Geometry check sheet. Reference: the model listing, model coordinates, mm. A direction names the side the tool comes from. Coordinates: 2 decimals unless noted, no trailing zeros. Write each loop counter-clockwise with the first axis right and the second up, starting at its lowest first coordinate (ties: lowest second). Pieces come first, ordered by that corner, then holes. Notation, with made-up numbers: (-11, 40) -> (-7, 40) arc R26 cw to (-7, 56) -> close; hole circle Ø5 at (-2, -30). An arc over 180 degrees is marked (long way). Answer in a Markdown table with one row per item. Add a question column.
1. Mould release check, pull along Z, two halves, no side actions. Record for faces 1 (the flat face through (6, 28.05, 35)), 2 (the flat face through (2, 14, 26)), 3 (the flat face through (8.9, 5.8, -18.2)): pulls with the +Z half, pulls with the -Z half, needs draft (parallel to the pull), parting line crosses it, or undercut.
2. Set-up check for faces 4 (the flat face through (6, 24.5, 35)), 5 (the flat face through (0, 10, 0)), 6 (the flat face through (6, 31, -46)), 7 (the cylindrical face through (5.9, 31.2, 40.5)), 8 (the flat face through (7.67, 8.09, 18.41)): record each of +Z, -Z, +X, -X, +Y, -Y from which the full face is reachable in a straight line by a thin tool's end or side.
3. Depth check by flat-ended pin: P1, Ø0.8, axis at x = 5.5, z = -34.5, coming from the -Y side; P2, Ø5.5, axis at y = 10, z = -5, coming from the +X side; P3, Ø6, axis at y = 28, z = -17, coming from the +X side. Enter the tip coordinate at first touch or a pass-through.
4. Cross-section at B-B on y = 21.5. Record the cut outline in (x, z), and give its area (3 significant figures).
5. Scan lines: L1, parallel to Z at x = 8, y = 9; L2, parallel to Y at x = 6.5, z = 37; L3, parallel to X at y = 19, z = -5.5. Record each from-to range of solid material in increasing order. Write a range as from..to.
```python
from build123d import *

# Parameters (mm, degrees)
BOSS_EXTRUDE1_DEPTH = 46
CUT_EXTRUDE1_REACH  = 62.101
SKETCH2_W           = 20
SKETCH2_H           = 24.5
FILLET1_R           = 2
FILLET2_R           = 4
CUT_EXTRUDE2_REACH  = 62.101
SKETCH4_R           = 4.3
BOSS_EXTRUDE2_DEPTH = 1.3
SKETCH5_R           = 4.25
BOSS_EXTRUDE3_DEPTH = 5
CHAMFER1_SIZE       = 0.3
CUT_EXTRUDE3_DEPTH  = 2.5


with BuildPart() as part:
    # Sketch1 → Boss-Extrude1 (new, symmetric)
    with BuildSketch(Plane.XY):
        with BuildLine():
            Line((0, 0), (2.6, 0))
            Line((2.6, 0), (2.6, 19))
            ThreePointArc((2.6, 19), (2.892893219, 19.707106781), (3.6, 20))
            Line((3.6, 20), (3.618034897, 20))
            ThreePointArc((3.618034897, 20), (6.16361931, 21.054415588), (7.218034897, 23.6))
            Line((7.218034897, 23.6), (7.218034897, 38))
            Line((7.218034897, 38), (4.618034897, 38))
            Line((4.618034897, 38), (4.618034897, 23.6))
            ThreePointArc((4.618034897, 23.6), (4.325141678, 22.892893219), (3.618034897, 22.6))
            Line((3.618034897, 22.6), (3.6, 22.6))
            ThreePointArc((3.6, 22.6), (1.054415588, 21.545584412), (0, 19))
            Line((0, 19), (0, 0))
        make_face()
    extrude(amount=BOSS_EXTRUDE1_DEPTH, both=True)

    # Sketch2 → Cut-Extrude1 (cut, up to next)
    with BuildSketch(Plane(origin=(7.218034897, 0, 0), x_dir=(0, 0, -1), z_dir=(1, 0, 0)), mode=Mode.PRIVATE) as cut_extrude1_sk1:
        with Locations((-36, 12.25)):
            Rectangle(SKETCH2_W, SKETCH2_H)
    cut_extrude1_tool1 = extrude(cut_extrude1_sk1.sketch, amount=-CUT_EXTRUDE1_REACH, mode=Mode.PRIVATE) & part.part
    # Sketch2 → Cut-Extrude1 (cut, up to next)
    with BuildSketch(Plane(origin=(7.218034897, 0, 0), x_dir=(0, 0, -1), z_dir=(1, 0, 0)), mode=Mode.PRIVATE) as cut_extrude1_sk2:
        with Locations((36, 12.25)):
            Rectangle(SKETCH2_W, SKETCH2_H)
    cut_extrude1_tool2 = extrude(cut_extrude1_sk2.sketch, amount=-CUT_EXTRUDE1_REACH, mode=Mode.PRIVATE) & part.part
    add(cut_extrude1_tool1.solids().sort_by_distance((7.218035, 12.25, 36))[0], mode=Mode.SUBTRACT)
    add(cut_extrude1_tool2.solids().sort_by_distance((7.218035, 12.25, -36))[0], mode=Mode.SUBTRACT)

    # Fillet1
    fillet1_edges = [part.edges().sort_by_distance(p)[0] for p in [
        (5.918034897, 38, -46),
        (5.918034897, 38, 46),
        (5.918034897, 24.5, 46),
        (5.918034897, 24.5, -46),
    ]]
    fillet(fillet1_edges, radius=FILLET1_R)

    # Fillet2
    fillet2_edges = [part.edges().sort_by_distance(p)[0] for p in [
        (1.3, 0, 26),
        (1.3, 0, -26),
    ]]
    fillet(fillet2_edges, radius=FILLET2_R)

    # Sketch3 → Cut-Extrude2 (cut, up to next)
    with BuildSketch(Plane(origin=(7.218034897, 0, 0), x_dir=(0, 0, -1), z_dir=(1, 0, 0)), mode=Mode.PRIVATE) as cut_extrude2_sk1:
        with BuildLine():
            Line((-37.25, 34.55), (-33.25, 34.55))
            ThreePointArc((-33.25, 34.55), (-30, 31.3), (-33.25, 28.05))
            Line((-33.25, 28.05), (-37.25, 28.05))
            ThreePointArc((-37.25, 28.05), (-40.5, 31.3), (-37.25, 34.55))
        make_face()
    cut_extrude2_tool1 = extrude(cut_extrude2_sk1.sketch, amount=-CUT_EXTRUDE2_REACH, mode=Mode.PRIVATE) & part.part
    # Sketch3 → Cut-Extrude2 (cut, up to next)
    with BuildSketch(Plane(origin=(7.218034897, 0, 0), x_dir=(0, 0, -1), z_dir=(1, 0, 0)), mode=Mode.PRIVATE) as cut_extrude2_sk2:
        with BuildLine():
            Line((37.25, 34.55), (33.25, 34.55))
            ThreePointArc((33.25, 34.55), (30, 31.3), (33.25, 28.05))
            Line((33.25, 28.05), (37.25, 28.05))
            ThreePointArc((37.25, 28.05), (40.5, 31.3), (37.25, 34.55))
        make_face()
    cut_extrude2_tool2 = extrude(cut_extrude2_sk2.sketch, amount=-CUT_EXTRUDE2_REACH, mode=Mode.PRIVATE) & part.part
    add(cut_extrude2_tool1.solids().sort_by_distance((7.218035, 31.3, 35.25))[0], mode=Mode.SUBTRACT)
    add(cut_extrude2_tool2.solids().sort_by_distance((7.218035, 31.3, -35.25))[0], mode=Mode.SUBTRACT)

    # Sketch4 → Boss-Extrude2 (add)
    with BuildSketch(Plane(origin=(2.6, 0, 0), x_dir=(0, 0, -1), z_dir=(1, 0, 0))):
        with Locations(Location((-16.5, 7.5, 0), (0, 0, 180))):
            Circle(SKETCH4_R)
        with Locations(Location((16.5, 7.5, 0), (0, 0, 180))):
            Circle(SKETCH4_R)
    extrude(amount=BOSS_EXTRUDE2_DEPTH)

    # Sketch5 → Boss-Extrude3 (add)
    with BuildSketch(Plane(origin=(3.9, 0, 0), x_dir=(0, 0, -1), z_dir=(1, 0, 0))):
        with Locations((-16.5, 7.5)):
            Circle(SKETCH5_R)
        with Locations((16.5, 7.5)):
            Circle(SKETCH5_R)
    extrude(amount=BOSS_EXTRUDE3_DEPTH)

    # Chamfer1
    chamfer1_edges = [part.edges().sort_by_distance(p)[0] for p in [
        (8.9, 7.5, 20.75),
        (8.9, 7.5, -12.25),
    ]]
    chamfer(chamfer1_edges, length=CHAMFER1_SIZE)

    # Sketch6 → Cut-Extrude3 (cut)
    with BuildSketch(Plane(origin=(8.9, 0, 0), x_dir=(0, 0, -1), z_dir=(1, 0, 0))):
        Polygon((-14.916307537, 5.819151549), (-14.25249631, 8.03109368), (-15.836188773, 9.711942131), (-18.083692463, 9.180848451), (-18.74750369, 6.96890632), (-17.163811227, 5.288057869), align=None)
        Polygon((14.946369576, 5.791326293), (17.202939625, 5.300179731), (18.756570049, 7.008853438), (18.053630424, 9.208673707), (15.797060375, 9.699820269), (14.243429951, 7.991146562), align=None)
    extrude(amount=-CUT_EXTRUDE3_DEPTH, mode=Mode.SUBTRACT)


solid = part.part
```
Results found:
| question | item | result |
|---|---|---|
| 1 | face 1 | undercut |
| 1 | face 2 | pulls with the +Z half |
| 1 | face 3 | needs draft |
| 2 | face 4 | +Z, +X, -X, -Y |
| 2 | face 5 | +Z, -Z, -X, +Y, -Y |
| 2 | face 6 | -Z, +X, -X, +Y, -Y |
| 2 | face 7 | +X, -X |
| 2 | face 8 | +X |
| 3 | P1 | stops at y = 24.5 |
| 3 | P2 | stops at x = 2.6 |
| 3 | P3 | stops at x = 7.22 |
| 4 | outline | (1.01, -26) -> (6.54, -26) -> (6.54, 26) -> (1.01, 26) -> close |
| 4 | area | 288 mm^2 |
| 5 | L1 | z = -20.48..-18.12, -15.16..-12.52, 12.52..15.17, 18.14..20.48 |
| 5 | L2 | y = 24.5..28.05, 34.55..38 |
| 5 | L3 | x = 0..2.6 |
